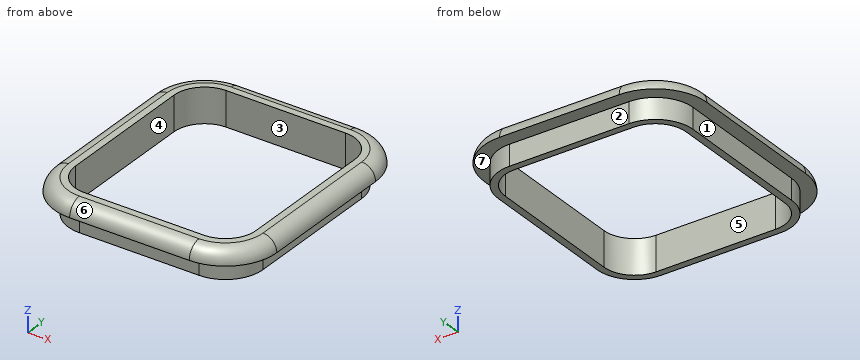
from build123d import *

# Parameters (mm, degrees)
F1_DEPTH = 15
F2_DEPTH = 10
F3_R     = 9.99999


# Not quite as in the source:
# - a fillet or chamfer is up to 0.001 mm smaller than in the source, because OpenCascade refuses the exact size
# - a feature of the source that left no trace in its solid (it failed there, or was rolled back) is left out


with BuildPart() as f1:
    # F0 (on Top) → F1 (new body)
    with BuildSketch(Plane.XY):
        with BuildLine():
            Line((-43, -77.5), (43, -77.5))
            ThreePointArc((43, -77.5), (62.091883092, -69.591883092), (70, -50.5))
            Line((70, -50.5), (70, 50.5))
            ThreePointArc((70, 50.5), (62.091883092, 69.591883092), (43, 77.5))
            Line((43, 77.5), (-43, 77.5))
            ThreePointArc((-43, 77.5), (-62.091883092, 69.591883092), (-70, 50.5))
            Line((-70, 50.5), (-70, -50.5))
            ThreePointArc((-70, -50.5), (-62.091883092, -69.591883092), (-43, -77.5))
        make_face()
        with BuildLine():
            Line((64.9999988648, 50.5), (64.9999988648, -50.5))
            ThreePointArc((64.9999988648, -50.5), (58.5563483834, -66.0563483834), (43, -72.4999988648))
            Line((43, -72.4999988648), (-43, -72.4999988648))
            ThreePointArc((-43, -72.4999988648), (-58.5563483834, -66.0563483834), (-64.9999988648, -50.5))
            Line((-64.9999988648, -50.5), (-64.9999988648, 50.5))
            ThreePointArc((-64.9999988648, 50.5), (-58.5563483834, 66.0563483834), (-43, 72.4999988648))
            Line((-43, 72.4999988648), (43, 72.4999988648))
            ThreePointArc((43, 72.4999988648), (58.5563483834, 66.0563483834), (64.9999988648, 50.5))
        make_face(mode=Mode.SUBTRACT)
    extrude(amount=-F1_DEPTH)

    # F0 (on Top) → F2 (join)
    with BuildSketch(Plane.XY):
        with BuildLine():
            Line((80, -50.5), (80, 50.5))
            ThreePointArc((80, 50.5), (69.1629509039, 76.6629509039), (43, 87.5))
            Line((43, 87.5), (-43, 87.5))
            ThreePointArc((-43, 87.5), (-69.1629509039, 76.6629509039), (-80, 50.5))
            Line((-80, 50.5), (-80, -50.5))
            ThreePointArc((-80, -50.5), (-69.1629509039, -76.6629509039), (-43, -87.5))
            Line((-43, -87.5), (43, -87.5))
            ThreePointArc((43, -87.5), (69.1629509039, -76.6629509039), (80, -50.5))
        make_face()
        with BuildLine():
            ThreePointArc((70, -50.5), (62.091883092, -69.591883092), (43, -77.5))
            Line((43, -77.5), (-43, -77.5))
            ThreePointArc((-43, -77.5), (-62.091883092, -69.591883092), (-70, -50.5))
            Line((-70, -50.5), (-70, 50.5))
            ThreePointArc((-70, 50.5), (-62.091883092, 69.591883092), (-43, 77.5))
            Line((-43, 77.5), (43, 77.5))
            ThreePointArc((43, 77.5), (62.091883092, 69.591883092), (70, 50.5))
            Line((70, 50.5), (70, -50.5))
        make_face(mode=Mode.SUBTRACT)
        with BuildLine():
            Line((-43, -77.5), (43, -77.5))
            ThreePointArc((43, -77.5), (62.091883092, -69.591883092), (70, -50.5))
            Line((70, -50.5), (70, 50.5))
            ThreePointArc((70, 50.5), (62.091883092, 69.591883092), (43, 77.5))
            Line((43, 77.5), (-43, 77.5))
            ThreePointArc((-43, 77.5), (-62.091883092, 69.591883092), (-70, 50.5))
            Line((-70, 50.5), (-70, -50.5))
            ThreePointArc((-70, -50.5), (-62.091883092, -69.591883092), (-43, -77.5))
        make_face()
        with BuildLine():
            Line((64.9999988648, 50.5), (64.9999988648, -50.5))
            ThreePointArc((64.9999988648, -50.5), (58.5563483834, -66.0563483834), (43, -72.4999988648))
            Line((43, -72.4999988648), (-43, -72.4999988648))
            ThreePointArc((-43, -72.4999988648), (-58.5563483834, -66.0563483834), (-64.9999988648, -50.5))
            Line((-64.9999988648, -50.5), (-64.9999988648, 50.5))
            ThreePointArc((-64.9999988648, 50.5), (-58.5563483834, 66.0563483834), (-43, 72.4999988648))
            Line((-43, 72.4999988648), (43, 72.4999988648))
            ThreePointArc((43, 72.4999988648), (58.5563483834, 66.0563483834), (64.9999988648, 50.5))
        make_face(mode=Mode.SUBTRACT)
    extrude(amount=F2_DEPTH)

    # F3 (radius 10 in the source; OpenCascade refuses exactly that, so slightly less here)
    f3_edges = [f1.edges().sort_by_distance(p)[0] for p in [
        (-69.162951, -76.662951, 10),
        (80, 0, 10),
        (69.162951, 76.662951, 10),
        (0, 87.5, 10),
        (-69.162951, 76.662951, 10),
        (-80, 0, 10),
        (0, -87.5, 10),
        (69.162951, -76.662951, 10),
    ]]
    fillet(f3_edges, radius=F3_R)


solid = f1.part
Input: part model. Units: mm. Frame: model coordinates. Face numbers are marked on the shaded views. A direction names the side the tool comes from. Round coordinates to 2 decimals unless told otherwise and drop trailing zeros. Loops run counter-clockwise (first coordinate to the right, second up) from the corner with the lowest first, then second, coordinate; pieces in that order, holes last. Notation, with made-up numbers: (14.25, 21) -> (65.25, 21) arc R23 ccw to (65.25, 36) -> close; hole circle Ø5 at (-7.75, 74.5). An arc over 180 degrees is marked (long way). Answer as a JSON object with one key per item and string values. Group by question number.
1) Pin query (flat end, axial travel): pin 1 (10 mm diameter, centred on x = -55.5, y = -28.5, fed in from +Z); pin 2 (4.5 mm diameter, centred on y = 10, z = -6.5, fed in from +X); pin 3 (12 mm diameter, centred on y = -63, z = 2, fed in from -X); pin 4 (12.5 mm diameter, centred on x = 8, z = -7, fed in from +Y). Return the tip coordinate at first contact, or that it passes through.
2) Reachability of the marked faces 1, 2 and 3 from +Z, -Z, +X, -X, +Y, -Y: full face, straight path, thin tool, end or side. Return the list, or none.
3) Section query D-D on z = 6.25. Output: boundary loops of the cut face in (x, y).
4) Section query C-C on z = -5. Output: boundary loops of the cut face in (x, y).
5) Ray query, L1, parallel to X at y = 34, z = 0.5; L2, parallel to X at y = -32.5, z = -13; L3, parallel to Y at x = -1, z = -12.5. Return the intervals inside material, ascending.
6) Draft query along Y for the marked faces 4, 5, 6 and 7. Return one class per face: +Y half, -Y half, draft (parallel to the pull), parting line (faces both ways), or undercut.
Reply:
{
 "1": {"pin 1": "passes through", "pin 2": "stops at x = 70", "pin 3": "stops at x = -79.38", "pin 4": "stops at y = 77.5"},
 "2": {"face 1": "-Z, -X, +Y, -Y", "face 2": "-Z, +X, -X, +Y", "face 3": "+Z, -Z"},
 "3": {"outline": "(-77.81, -50.5) arc R34.81 ccw to (-43, -85.31) -> (43, -85.31) arc R34.81 ccw to (77.81, -50.5) -> (77.81, 50.5) arc R34.81 ccw to (43, 85.31) -> (-43, 85.31) arc R34.81 ccw to (-77.81, 50.5) -> close; hole (-65, -50.5) arc R22 ccw to (-43, -72.5) -> (43, -72.5) arc R22 ccw to (65, -50.5) -> (65, 50.5) arc R22 ccw to (43, 72.5) -> (-43, 72.5) arc R22 ccw to (-65, 50.5) -> close"},
 "4": {"outline": "(-70, -50.5) arc R27 ccw to (-43, -77.5) -> (43, -77.5) arc R27 ccw to (70, -50.5) -> (70, 50.5) arc R27 ccw to (43, 77.5) -> (-43, 77.5) arc R27 ccw to (-70, 50.5) -> close; hole (-65, -50.5) arc R22 ccw to (-43, -72.5) -> (43, -72.5) arc R22 ccw to (65, -50.5) -> (65, 50.5) arc R22 ccw to (43, 72.5) -> (-43, 72.5) arc R22 ccw to (-65, 50.5) -> close"},
 "5": {"L1": "x = -79.99 to -65, 65 to 79.99", "L2": "x = -70 to -65, 65 to 70", "L3": "y = -77.5 to -72.5, 72.5 to 77.5"},
 "6": {"face 4": "undercut", "face 5": "undercut", "face 6": "-Y half", "face 7": "draft"}
}
